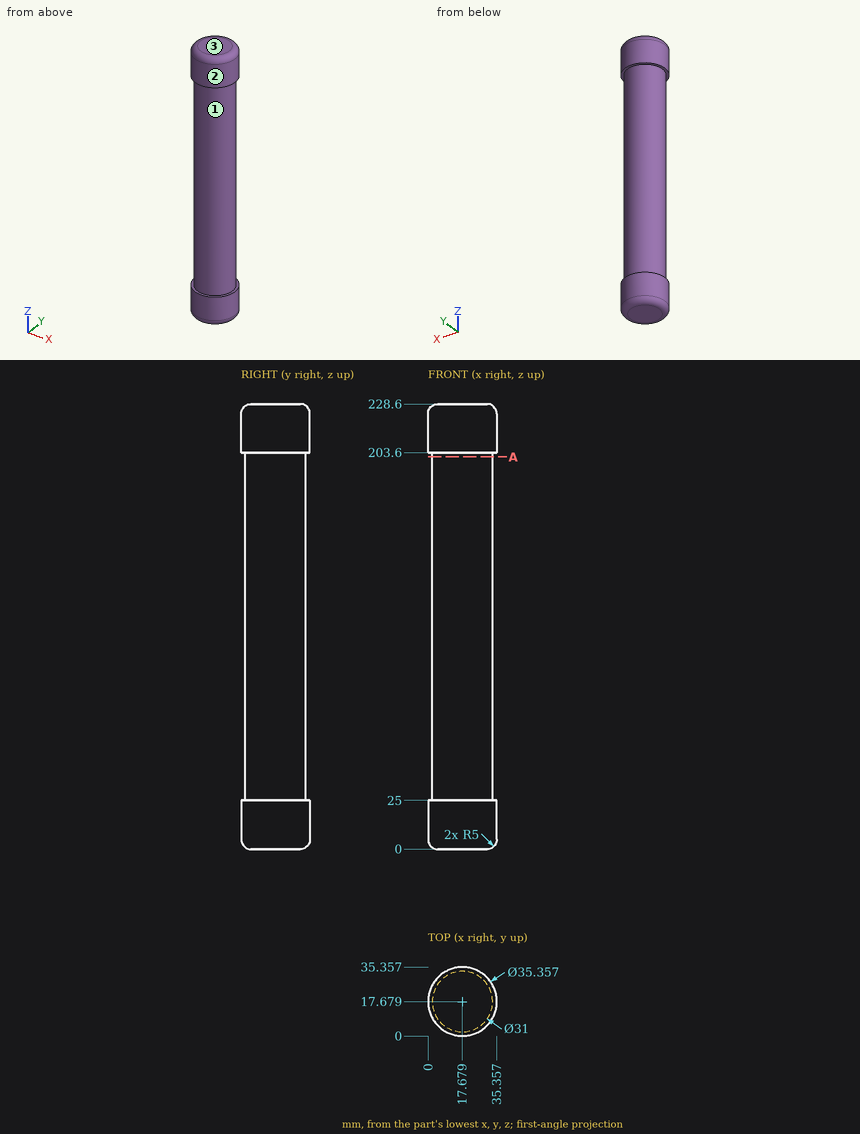
The figure shows three views and two pictorial views of one solid part (mm, origin at its lowest corner). Answer the questions. Round coordinates to 2 decimals unless told otherwise and drop trailing zeros. Order: outer loops, then holes, each group sorted by start corner. A loop starts at its lowest first (then second) coordinate and runs counter-clockwise, first axis right, second up. Notation, with made-up numbers: M 17.25,33 L 68.25,33 A18 ccw 68.25,48 Z; hole C -18,-26.75 d3. An arc over 180 degrees is marked long. Answer in a Markdown table with one row per item. Add a question column.
1) Flat-ended cylindrical pins translate along their axes: pin 1 Ø6 at (y, z) = (30, 161) entering from -X (1 decimal); pin 2 Ø8 at (y, z) = (23, 25) entering from +X; pin 3 Ø3 at (x, z) = (29.5, 37) entering from -Y (1 decimal). Find the tip coordinate at first contact, or state that the pin passes through.
2) Determine the mould class of the marked faces 1, 2 and 3 for opening direction Z: pulls with the +Z half, pulls with the -Z half, needs draft (parallel to the pull), parting line crosses it, or undercut.
3) The part is cut by section A-A on z = 201.5. Determine the outline of the cut face in (x, y), plus the area to 3 significant figures.
4) Consider line 1 along X through (y, z) = (17, 126.5); line 2 along X through (y, z) = (21, 177); line 3 along Z through (x, y) = (27.5, 30). Determine where each line is inside the solid, lowest interval first. Write a range as from..to.
Findings below:
| question | item | result |
|---|---|---|
| 1 | pin 1 | stops at x = 5.3 |
| 1 | pin 2 | stops at x = 35.31 |
| 1 | pin 3 | stops at y = 6.1 |
| 2 | face 1 | undercut |
| 2 | face 2 | needs draft |
| 2 | face 3 | pulls with the +Z half |
| 3 | outline | C 17.68,17.68 d31 |
| 3 | area | 755 mm² |
| 4 | line 1 | x = 2.19..33.16 |
| 4 | line 2 | x = 2.54..32.82 |
| 4 | line 3 | z = 1.06..25, 203.6..227.54 |
